Study the drawing (mm; zero at the part's minimum x, y, z) and answer. Coordinates: 2 decimals unless noted, no trailing zeros. Order: outer loops, then holes, each group sorted by start corner. A loop starts at its lowest first (then second) coordinate and runs counter-clockwise, first axis right, second up.
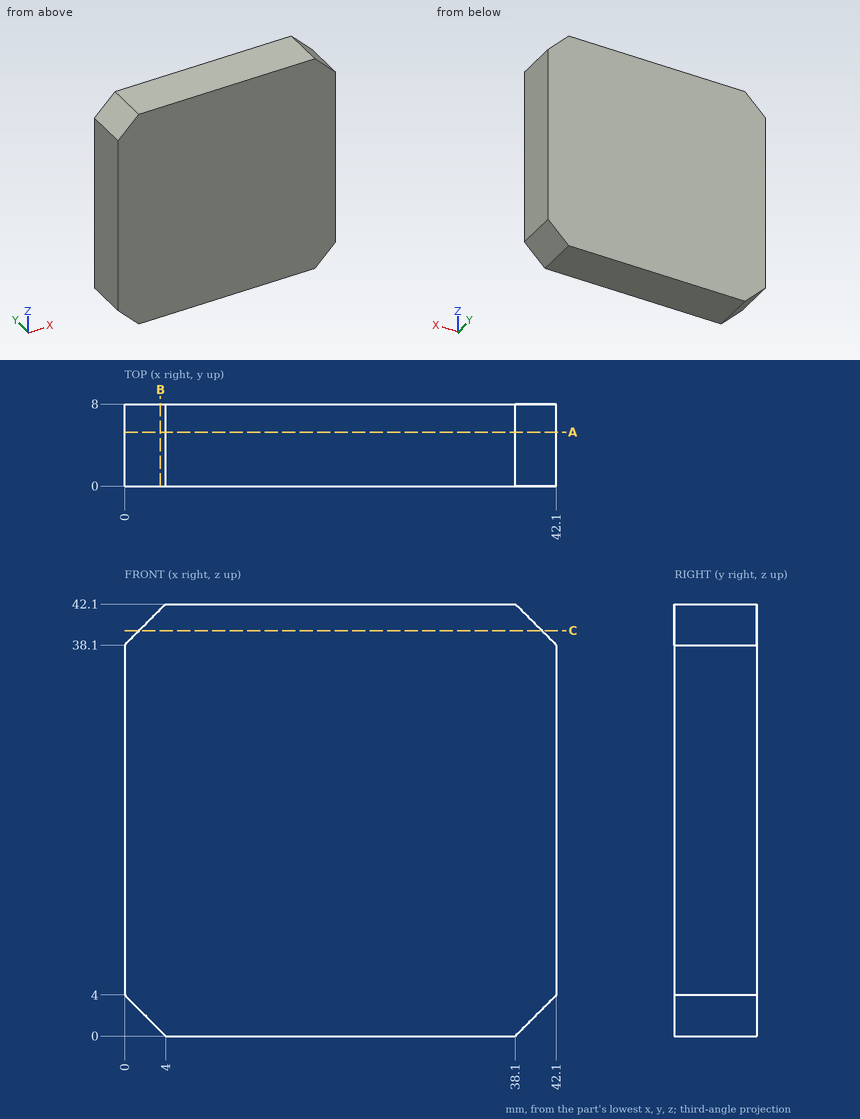
1) A cutting plane is placed at B-B, the plane x = 3.5. Determine the outline of the cut face in (y, z), and give its area (3 significant figures).
A:
outline: (0, 0.5) - (8, 0.5) - (8, 41.6) - (0, 41.6) - close
area: 329 mm2
2) A cutting plane is placed at A-A, the plane y = 5.25. Determine the outline of the cut face in (x, z), and give its area (3 significant figures).
A:
outline: (0, 4) - (4, 0) - (38.1, 0) - (42.1, 4) - (42.1, 38.1) - (38.1, 42.1) - (4, 42.1) - (0, 38.1) - close
area: 1,740 mm2
3) Straight lines are drawn through the part: line 1 (Z direction, x = 2.5, y = 2.5); line 2 (Z direction, x = 3, y = 4.75); line 3 (X direction, y = 1.25, z = 2). For each, find the intervals that lie inside material, in ascending order.
A:
line 1: z = 1.5 to 40.6
line 2: z = 1 to 41.1
line 3: x = 2 to 40.1
4) A cutting plane is placed at C-C, the plane z = 39.5. Determine the outline of the cut face in (x, y), and give its area (3 significant figures).
A:
outline: (1.4, 0) - (40.7, 0) - (40.7, 8) - (1.4, 8) - close
area: 314 mm2
